Could you check a few things on this model? Use its own coordinates, in mm. Face numbers are marked on the shaded views. A direction names the side the tool comes from. Coordinates: 2 decimals unless noted, no trailing zeros. Write each loop counter-clockwise with the first axis right and the second up, starting at its lowest first coordinate (ties: lowest second). Pieces come first, ordered by that corner, then holes.
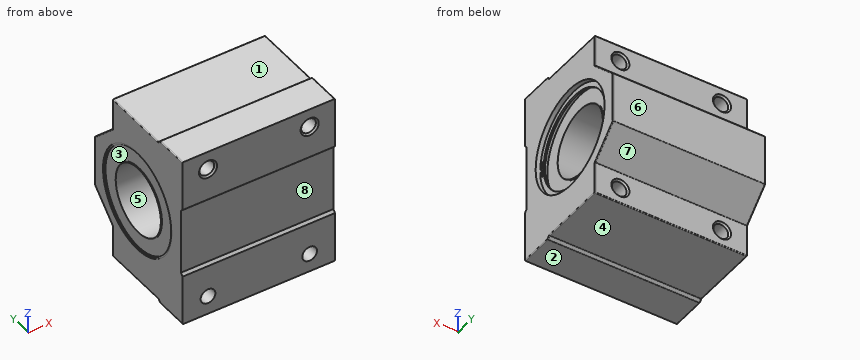
```python
from build123d import *

# Parameters (mm, degrees)
SKETCH1_R           = 30.5
BOSS_EXTRUDE1_DEPTH = 90
EXTRUDE_THIN1_START = 0.5
SKETCH1_4_R         = 20.5
SKETCH1_4_R_2       = 20
EXTRUDE_THIN1_DEPTH = 83.5
BOSS_EXTRUDE2_START = 0.8
SKETCH1_5_R         = 29.5
SKETCH1_5_R_2       = 20
BOSS_EXTRUDE2_DEPTH = 83
BOSS_EXTRUDE3_START = 0.3
SKETCH1_6_R         = 30.5
SKETCH1_6_R_2       = 29.5
BOSS_EXTRUDE3_DEPTH = 85
BOSS_EXTRUDE4_START = 1
BOSS_EXTRUDE4_DEPTH = 1
FILLET1_R           = 0.5
SKETCH4_R           = 4.35
CUT_EXTRUDE3_DEPTH  = 130.55693729
CHAMFER1_SIZE       = 1


with BuildPart() as part:
    # Sketch1 → Boss-Extrude1 (new body)
    with BuildSketch(Plane(origin=(0, 0, 0), x_dir=(0, 0, -1), z_dir=(1, 0, 0))):
        Polygon((-51, -20), (-49.5, -18.5), (-49.5, 22), (-30.5, 22), (-15, 38), (15, 38), (30.5, 22), (49.5, 22), (49.5, -18.5), (51, -20), (51, -40), (21, -40), (19.5, -38.5), (-19.5, -38.5), (-21, -40), (-51, -40), align=None)
        with Locations(Location((0, 0, 0), (0, 0, 180))):
            Circle(SKETCH1_R, mode=Mode.SUBTRACT)
    extrude(amount=BOSS_EXTRUDE1_DEPTH)



with BuildPart() as body_2:
    # Sketch1_4 → Extrude-Thin1 (new body)
    with BuildSketch(Plane(origin=(0, 0, 0), x_dir=(0, 0, -1), z_dir=(1, 0, 0)).offset(EXTRUDE_THIN1_START)):
        Circle(SKETCH1_4_R)
        Circle(SKETCH1_4_R_2, mode=Mode.SUBTRACT)
    extrude(amount=EXTRUDE_THIN1_DEPTH)

    # Sketch1_5 → Boss-Extrude2 (add)
    with BuildSketch(Plane(origin=(0, 0, 0), x_dir=(0, 0, -1), z_dir=(1, 0, 0)).offset(BOSS_EXTRUDE2_START)):
        Circle(SKETCH1_5_R)
        with Locations(Location((0, 0, 0), (0, 0, 180))):
            Circle(SKETCH1_5_R_2, mode=Mode.SUBTRACT)
    extrude(amount=BOSS_EXTRUDE2_DEPTH)


with BuildPart() as part_1:
    add(part.part)

    add(body_2.part)  # Boss-Extrude3 merges body 2
    # Sketch1_6 → Boss-Extrude3 (add)
    with BuildSketch(Plane(origin=(0, 0, 0), x_dir=(0, 0, -1), z_dir=(1, 0, 0)).offset(BOSS_EXTRUDE3_START)):
        with Locations(Location((0, 0, 0), (0, 0, 180))):
            Circle(SKETCH1_6_R)
        Circle(SKETCH1_6_R_2, mode=Mode.SUBTRACT)
    extrude(amount=BOSS_EXTRUDE3_DEPTH)

    # Sketch3 → Boss-Extrude4 (add)
    with BuildSketch(Plane(origin=(85.3, 0, 0), x_dir=(0, 0, -1), z_dir=(1, 0, 0)).offset(BOSS_EXTRUDE4_START)):
        with BuildLine():
            Line((-1.001295059, -29.483002022), (-1.035237264, -30.482425819))
            ThreePointArc((-1.035237264, -30.482425819), (0, 30.5), (1.035237264, -30.482425819))
            Line((1.035237264, -30.482425819), (1.001295059, -29.483002022))
            ThreePointArc((1.001295059, -29.483002022), (1.67030528, -28.488037708), (2.813261111, -28.850226376))
            ThreePointArc((2.813261111, -28.850226376), (4.517048294, -28.723259657), (3.621379804, -27.268340668))
            ThreePointArc((3.621379804, -27.268340668), (0, 27.507758805), (-3.621379804, -27.268340668))
            ThreePointArc((-3.621379804, -27.268340668), (-4.517048294, -28.723259657), (-2.813261111, -28.850226376))
            ThreePointArc((-2.813261111, -28.850226376), (-1.67030528, -28.488037708), (-1.001295059, -29.483002022))
        make_face()
    extrude(amount=BOSS_EXTRUDE4_DEPTH)

    # Fillet1
    fillet1_edges = [part_1.edges().sort_by_distance(p)[0] for p in [
        (90, -19.25, 50.25),
        (90, -30, 51),
        (0, 1.75, 49.5),
        (0, 22, 40),
        (0, 30, 22.75),
        (0, 38, 0),
        (0, 30, -22.75),
        (0, 22, -40),
        (0, 1.75, -49.5),
        (0, -19.25, -50.25),
        (0, -30, -51),
        (0, -30, 51),
        (0, -19.25, 50.25),
        (45, -18.5, 49.5),
        (45, 22, 49.5),
        (45, 22, 30.5),
        (45, 38, 15),
        (45, 38, -15),
        (45, 22, -30.5),
        (45, 22, -49.5),
        (45, -18.5, -49.5),
        (45, -20, -51),
        (45, -20, 51),
        (90, -30, -51),
        (90, -19.25, -50.25),
        (90, 1.75, -49.5),
        (90, 22, -40),
        (90, 30, -22.75),
        (90, 38, 0),
        (90, 30, 22.75),
        (90, 22, 40),
        (90, 1.75, 49.5),
    ]]
    fillet(fillet1_edges, radius=FILLET1_R)

    # Sketch4 → Cut-Extrude3 (cut, through all)
    with BuildSketch(Plane.XZ.offset(40)):
        with Locations(Location((15, 40, 0), (0, 0, 270))):
            Circle(SKETCH4_R)
        with Locations(Location((75, 40, 0), (0, 0, 270))):
            Circle(SKETCH4_R)
        with Locations(Location((75, -40, 0), (0, 0, 270))):
            Circle(SKETCH4_R)
        with Locations(Location((15, -40, 0), (0, 0, 270))):
            Circle(SKETCH4_R)
    extrude(amount=-CUT_EXTRUDE3_DEPTH, mode=Mode.SUBTRACT)

    # Chamfer1
    chamfer1_edges = [part_1.edges().sort_by_distance(p)[0] for p in [
        (15, 22, -35.65),
        (75, 22, -35.65),
        (75, 22, 44.35),
        (75, -40, 44.35),
        (15, 22, 44.35),
        (15, -40, 44.35),
    ]]
    chamfer(chamfer1_edges, length=CHAMFER1_SIZE)


solid = part_1.part
```
1. I want a section at B-B on x = 26. Please give me the cut outline in (y, z).
Verdict:
outline: (-40, -51) - (-20.21, -51) arc R0.5 ccw to (-19.85, -50.85) - (-18.65, -49.65) arc R0.5 cw to (-18.29, -49.5) - (21.5, -49.5) arc R0.5 ccw to (22, -49) - (22, -30.71) arc R0.5 cw to (22.15, -30.35) - (37.85, -15.15) arc R0.5 ccw to (38, -14.79) - (38, 14.79) arc R0.5 ccw to (37.85, 15.15) - (22.15, 30.35) arc R0.5 cw to (22, 30.71) - (22, 49) arc R0.5 ccw to (21.5, 49.5) - (-18.29, 49.5) arc R0.5 cw to (-18.65, 49.65) - (-19.85, 50.85) arc R0.5 ccw to (-20.21, 51) - (-40, 51) - (-40, 21) - (-38.5, 19.5) - (-38.5, -19.5) - (-40, -21) - close; hole circle Ø40 at (0, 0)
2. I want a section at A-A on z = -40. Please give me the cut outline in (x, y).
Verdict:
outline: (0, -40) - (10.65, -40) - (10.65, 21) - (9.65, 22) - (0.5, 22) arc R0.5 ccw to (0, 21.5) - close; (19.35, -40) - (70.65, -40) - (70.65, 21) - (69.65, 22) - (20.35, 22) - (19.35, 21) - close; (79.35, -40) - (90, -40) - (90, 21.5) arc R0.5 ccw to (89.5, 22) - (80.35, 22) - (79.35, 21) - close
3. For pin 1 (2 mm diameter, centred on x = 52, z = 17, fed in from -Y); pin 2 (20 mm diameter, centred on x = 60, z = 42, fed in from +Y); pin 3 (3 mm diameter, centred on x = 10.5, y = -6, fed in from +Z), each with a flat end and sliding along its axis, tell me the tip position at first contact or that it passes through.
Verdict:
pin 1: stops at y = -38.5
pin 2: stops at y = 22
pin 3: stops at z = 49.5
4. I want a section at C-C on y = 0. Give the number of separate pieces and of enclosed holes in the cut face, plus the area to 3 significant figures.
Verdict:
separate pieces: 2
enclosed holes: 4
area: 4,940 mm2
5. On a 3-axis mill with a long thin cutter (end or side, diameter ignored), from which of +Z, -Z, +X, -X, +Y, -Y can I reach the whole of each face in a straight line? I mean the marked faces 1, 2, 3, 4 and 5. Say none if no direction works.
Verdict:
face 1: +Z, +X, -X, +Y
face 2: -Z, +X, -X, +Y, -Y
face 3: -X
face 4: -Z, +X, -X, +Y
face 5: +X, -X
6. Please list where these lines run through material, in increasing order: line 1 along X through (y, z) = (-1.5, 39.5); line 2 along Y through (x, z) = (82.5, 0.5); line 3 along X through (y, z) = (19.5, 43.5).
Verdict:
line 1: x = 0 to 10.68, 19.32 to 70.68, 79.32 to 90
line 2: y = -38.5 to -19.99, 19.99 to 38
line 3: x = 0 to 12.42, 17.58 to 72.42, 77.58 to 90
7. If we mould it in two halves opening along Z, with no side actions, what happens to the marked faces 6, 7 and 8? For each: pulls with the +Z half, pulls with the -Z half, needs draft (parallel to the pull), parting line crosses it, or undercut.
Verdict:
face 6: needs draft
face 7: pulls with the -Z half
face 8: undercut
